```python
from build123d import *

# Parameters (mm, degrees)
BOSS_EXTRUDE1_DEPTH  = 1.5875
FILLET2_DEPTH        = 1.5875
M4_CLEARANCE_HOLE1_D = 4.5


with BuildPart() as part:
    # Sketch1 → Boss-Extrude1 (new body)
    with BuildSketch(Plane.XY):
        with BuildLine():
            Line((27.5, 6), (-27.5, 6))
            Line((-27.5, 6), (-27.5, -6))
            Line((-27.5, -6), (27.5, -6))
            Line((27.5, -6), (49.436268592, -12.218533657))
            ThreePointArc((49.436268592, -12.218533657), (40.2, -4.45e-07), (49.436267736, 12.218533415))
            Line((49.436267736, 12.218533415), (27.5, 6))
        make_face()
    extrude(amount=BOSS_EXTRUDE1_DEPTH)

    # Fillet2: read off the stored shape, not the designer's step
    # Fillet2 outline → Fillet2 (cut)
    with BuildSketch(Plane.XY):
        with BuildLine():
            ThreePointArc((-27.5, 4.222), (-26.979235857, 5.479235857), (-25.722, 6))
            Line((-25.722, 6), (-27.5, 6))
            Line((-27.5, 6), (-27.5, 4.222))
        make_face()
        with BuildLine():
            ThreePointArc((-25.722, -6), (-26.979235857, -5.479235857), (-27.5, -4.222))
            Line((-27.5, -4.222), (-27.5, -6))
            Line((-27.5, -6), (-25.722, -6))
        make_face()
        with BuildLine():
            Line((49.436267736, 12.218533415), (40.292754575, 9.626513532))
            ThreePointArc((40.292754575, 9.626513532), (42.209860363, 8.969548331), (42.266383414, 6.943788468))
            ThreePointArc((42.266383414, 6.943788468), (45.374075159, 10.229880512), (49.436267736, 12.218533415))
        make_face()
        with BuildLine():
            ThreePointArc((49.436267736, -12.218533415), (45.374075159, -10.229880512), (42.266383413, -6.943788468))
            ThreePointArc((42.266383413, -6.943788468), (42.209860363, -8.969548331), (40.292754575, -9.626513532))
            Line((40.292754575, -9.626513532), (49.436267736, -12.218533415))
        make_face()
    extrude(amount=FILLET2_DEPTH, mode=Mode.SUBTRACT)

    # M4 Clearance Hole1 (through all)
    with Locations(Plane.XY.offset(1.5875)):
        with Locations((-17.778, 0), (12.221650814, 0)):
            Hole(M4_CLEARANCE_HOLE1_D / 2)


solid = part.part
```
The listing builds one solid part. Answer for the finished solid, in the listing's coordinates (mm). A direction names the side the tool comes from. Coordinates: 2 decimals unless noted, no trailing zeros. Loops run counter-clockwise (first coordinate to the right, second up) from the corner with the lowest first, then second, coordinate; pieces in that order, holes last. Notation, with made-up numbers: (-17, 38) - (0, 38) arc R10 ccw to (0, 55) - close; hole circle Ø1 at (2, 41). An arc over 180 degrees is marked (long way). Use a Markdown table: item, result. Add a question column.
1) The part is cut by section C-C, the plane x = 19. Give the vertices of the cut face in (y, z), and give its area (4 significant figures).
2) The part is cut by section B-B, the plane z = 0.75. Give the vertices of the cut face in (x, y), and give its area (3 significant figures).
3) The part is cut by section A-A, the plane y = 0. Give the vertices of the cut face in (x, z).
4) Given pin 1 (0.5 mm diameter, centred on x = 2, z = 0.5, fed in from +Y), flat-ended and moving along its own axis, determine where the tip first touches the part or whether it passes through.
5) Find the intervals of material crossed by line 1 (Y direction, x = -18, z = 1.1); line 2 (Y direction, x = 26, z = 0.55); line 3 (X direction, y = -1, z = 1.35), in increasing order.
6) The mould has two halves that part along Y. Classify faces 4 (the cylindrical face through (-26.97, -5.49, 0.78)), 5 (the cylindrical face through (42.192, 8.994, 0.783)), 6 (the flat face through (33.99, 7.84, 0.78)): released by +Y, released by -Y, zero draft, split by the parting line, or undercut.
7) For faces 1 (the cylindrical face through (-19.924, 0.676, 0.783)), 2 (the flat face through (1, -6, 1)), 3 (the flat face through (1, 6, 1)), determine the directions among +Z, -Z, +X, -X, +Y, -Y from which every point of the face is accessible in a straight line to the end or side of a thin tool.
Here are the results:
| question | item | result |
|---|---|---|
| 1 | outline | (-6, 0) - (6, 0) - (6, 1.59) - (-6, 1.59) - close |
| 1 | area | 19.05 mm^2 |
| 2 | outline | (-27.5, -4.22) arc R1.78 ccw to (-25.72, -6) - (27.5, -6) - (40.29, -9.63) arc R1.78 ccw to (42.27, -6.94) arc R12.7 cw to (42.27, 6.94) arc R1.78 ccw to (40.29, 9.63) - (27.5, 6) - (-25.72, 6) arc R1.78 ccw to (-27.5, 4.22) - close; hole circle Ø4.5 at (-17.78, 0); hole circle Ø4.5 at (12.22, 0) |
| 2 | area | 846 mm^2 |
| 3 | outline | (-27.5, 0) - (-20.03, 0) - (-20.03, 1.59) - (-27.5, 1.59) - close; (-15.53, 0) - (9.97, 0) - (9.97, 1.59) - (-15.53, 1.59) - close; (14.47, 0) - (40.2, 0) - (40.2, 1.59) - (14.47, 1.59) - close |
| 4 | pin 1 | stops at y = 6 |
| 5 | line 1 | y = -6 to -2.24, 2.24 to 6 |
| 5 | line 2 | y = -6 to 6 |
| 5 | line 3 | x = -27.5 to -19.79, -15.76 to 10.21, 14.24 to 40.24 |
| 6 | face 4 | released by -Y |
| 6 | face 5 | undercut |
| 6 | face 6 | released by +Y |
| 7 | face 1 | +Z, -Z |
| 7 | face 2 | +Z, -Z, -X, -Y |
| 7 | face 3 | +Z, -Z, -X, +Y |
